from build123d import *

# Parameters (mm, degrees)
F0_R     = 21.881229
F1_DEPTH = 40
F2_SIZE  = 5
F3_R     = 5


with BuildPart() as f1:
    # F0 (on Front) → F1 (new body)
    with BuildSketch(Plane.XZ):
        Circle(F0_R)
    extrude(amount=F1_DEPTH)

    # F2
    f2_edges = [f1.edges().sort_by_distance(p)[0] for p in [
        (-21.881229, -40, 0),
    ]]
    chamfer(f2_edges, length=F2_SIZE)

    # F3
    f3_edges = [f1.edges().sort_by_distance(p)[0] for p in [
        (-21.881229, 0, 0),
    ]]
    fillet(f3_edges, radius=F3_R)


solid = f1.part
The model under review builds one solid part; all positions refer to its coordinate system, in mm. Round coordinates to 2 decimals unless told otherwise and drop trailing zeros. Write each loop counter-clockwise with the first axis right and the second up, starting at its lowest first coordinate (ties: lowest second). Pieces come first, ordered by that corner, then holes. Notation, with made-up numbers: M 41,23 L 72,23 A32 cw 72,55 Z; hole C 14.5,58.5 d1. An arc over 180 degrees is marked long. Use a Markdown table: item, result. Add a question column.
Q1. We need section A-A, the plane x = 0. State the section outline as (y, z) points, plus the area to 3 significant figures.
Q2. We need section D-D, the plane y = -3. State the section outline as (x, z) points.
Q3. To check wall thickness, follow line 1 (X direction, y = -11.5, z = -0.5); line 2 (Y direction, x = 1, z = 17); line 3 (Z direction, x = 15.5, y = -33). State the ranges of each line that lie inside material, in increasing order.
Q4. We need section C-C, the plane y = -22. State the section outline as (x, z) points.
Q5. Insertion check: pin 1 (6 mm diameter, centred on x = 9, y = -8.5, fed in from +Z); pin 2 (8 mm diameter, centred on y = -10.5, z = 5.5, fed in from -X); pin 3 (1 mm diameter, centred on y = -14, z = -6, fed in from +X); pin 4 (12 mm diameter, centred on y = -10.5, z = -2, fed in from +X). Each pin has a flat end and moves straight along its axis. Give the tip position at first contact, or say it passes through.
Q6. We need section B-B, the plane z = 0. State the section outline as (x, y) points, plus the area to 3 significant figures.
Findings below:
| question | item | result |
|---|---|---|
| 1 | outline | M -40,-16.88 L -35,-21.88 L -5,-21.88 A5 ccw 0,-16.88 L 0,16.88 A5 ccw -5,21.88 L -35,21.88 L -40,16.88 Z |
| 1 | area | 1,710 mm² |
| 2 | outline | C 0,0 d42.93 |
| 3 | line 1 | x = -21.88 to 21.88 |
| 3 | line 2 | y = -39.85 to 0 |
| 3 | line 3 | z = -15.44 to 15.44 |
| 4 | outline | C 0,0 d43.76 |
| 5 | pin 1 | stops at z = 21.04 |
| 5 | pin 2 | stops at x = -21.83 |
| 5 | pin 3 | stops at x = 21.18 |
| 5 | pin 4 | stops at x = 21.88 |
| 6 | outline | M -21.88,-35 L -16.88,-40 L 16.88,-40 L 21.88,-35 L 21.88,-5 A5 ccw 16.88,0 L -16.88,0 A5 ccw -21.88,-5 Z |
| 6 | area | 1,710 mm² |
